Could you check a few things on this drawing? It's one solid part, dimensions in mm from its lowest x, y, z. A direction names the side the tool comes from. Give positions to 0.01 mm unless a question says otherwise; leave off trailing zeros. Loops run counter-clockwise (first coordinate to the right, second up) from the corner with the lowest first, then second, coordinate; pieces in that order, holes last. Notation, with made-up numbers: (31, 83.5) - (82, 83.5) arc R20 ccw to (82, 103.5) - close; hole circle Ø10 at (30, 36). An arc over 180 degrees is marked (long way). Answer as a JSON object with one key per item and string values.
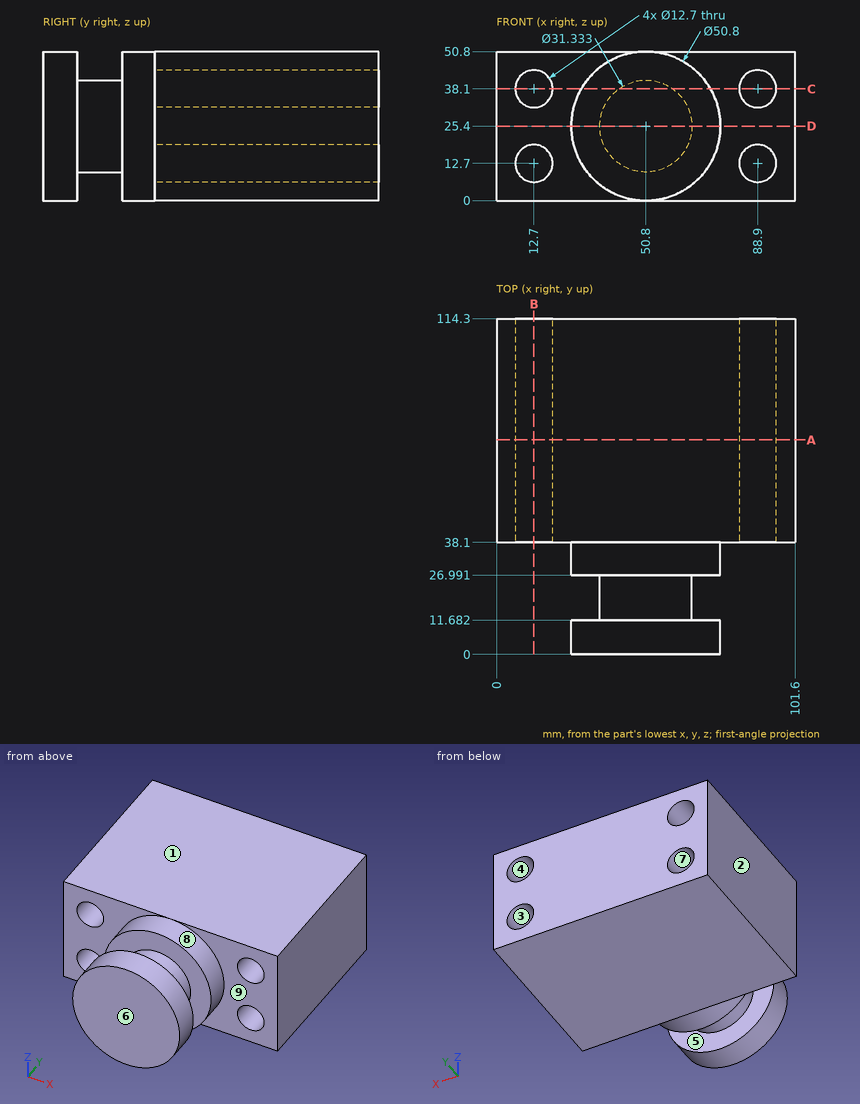
1) Imagine slicing it at A-A on y = 73. Write out the boundary of the cut face in (x, z), and give its area (3 significant figures).
Check sheet entries:
{"outline": "(0, 0) - (101.6, 0) - (101.6, 50.8) - (0, 50.8) - close; hole circle Ø12.7 at (12.7, 12.7); hole circle Ø12.7 at (12.7, 38.1); hole circle Ø12.7 at (88.9, 12.7); hole circle Ø12.7 at (88.9, 38.1)", "area": "4,650 mm2"}
2) Imagine slicing it at D-D on z = 25.4. Write out the boundary of the cut face in (x, y), and give its area (3 significant figures).
Check sheet entries:
{"outline": "(0, 38.1) - (25.4, 38.1) - (25.4, 26.99) - (35.13, 26.99) - (35.13, 11.68) - (25.4, 11.68) - (25.4, 0) - (76.2, 0) - (76.2, 11.68) - (66.47, 11.68) - (66.47, 26.99) - (76.2, 26.99) - (76.2, 38.1) - (101.6, 38.1) - (101.6, 114.3) - (0, 114.3) - close", "area": "9,380 mm2"}
3) If we mould it in two halves opening along Z, with no side actions, what happens to the marked faces 1, 2, 3 and 4? For each: released by +Z, released by -Z, zero draft, split by the parting line, or undercut.
Check sheet entries:
{"face 1": "released by +Z", "face 2": "zero draft", "face 3": "undercut", "face 4": "undercut"}
4) I'm going to push flat-ended pins straight in: P1, Ø6, axis at y = 18.5, z = 10.5, coming from the +X side; P2, Ø14.5, axis at x = 88.9, z = 38.1, coming from the -Y side; P3, Ø14.5, axis at x = 12.7, z = 12.7, coming from the +Y side; P4, Ø1, axis at y = 25, z = 40, coming from the +X side. Where does each tip first touch, or does it pass through?
Check sheet entries:
{"P1": "x = 60.99", "P2": "y = 38.1", "P3": "y = 114.3", "P4": "x = 57.63"}
5) Which directions (+Z, -Z, +X, -X, +Y, -Y) give clear straight access to the entire face, cutting with the end or side of a thin tool? Please do the marked faces 5, 6, 7, 8 and 9.
Check sheet entries:
{"face 5": "none", "face 6": "+Z, -Z, +X, -X, -Y", "face 7": "+Y, -Y", "face 8": "-Y", "face 9": "+X, -Y"}
6) Imagine slicing it at B-B on x = 12.7. Write out the boundary of the cut face in (y, z).
Check sheet entries:
{"outline": "(38.1, 0) - (114.3, 0) - (114.3, 6.35) - (38.1, 6.35) - close; (38.1, 19.05) - (114.3, 19.05) - (114.3, 31.75) - (38.1, 31.75) - close; (38.1, 44.45) - (114.3, 44.45) - (114.3, 50.8) - (38.1, 50.8) - close"}
7) I need wall thicknesses on L1, parallel to Z at x = 88.9, y = 78; L2, parallel to X at y = 62, z = 13; L3, parallel to X at y = 42.5, z = 18 (1 decimal). Which ranges of each line are inside material? Lowest first, please.
Check sheet entries:
{"L1": "0 to 6.35, 19.05 to 31.75, 44.45 to 50.8", "L2": "0 to 6.36, 19.04 to 82.56, 95.24 to 101.6", "L3": "0 to 9.2, 16.2 to 85.4, 92.4 to 101.6"}
8) Imagine slicing it at C-C on z = 38.1. Write out the boundary of the cut face in (x, y).
Check sheet entries:
{"outline": "(0, 38.1) - (6.35, 38.1) - (6.35, 114.3) - (0, 114.3) - close; (19.05, 38.1) - (28.8, 38.1) - (28.8, 26.99) - (41.63, 26.99) - (41.63, 11.68) - (28.8, 11.68) - (28.8, 0) - (72.8, 0) - (72.8, 11.68) - (59.97, 11.68) - (59.97, 26.99) - (72.8, 26.99) - (72.8, 38.1) - (82.55, 38.1) - (82.55, 114.3) - (19.05, 114.3) - close; (95.25, 38.1) - (101.6, 38.1) - (101.6, 114.3) - (95.25, 114.3) - close"}
